Autodesk Inventor part; units mm, degrees
ref_plane "YZ Plane" through (0, 0, 0) normal (1, 0, 0) x (0, 1, 0)
ref_plane "XZ Plane" through (0, 0, 0) normal (0, 1, 0) x (-1, 0, 0)
ref_plane "XY Plane" through (0, 0, 0) normal (0, 0, 1) x (1, 0, 0)
sketch "Sketch1" plane through (0, 0, 0) normal (0, 0, 1) x (1, 0, 0)
  line L0 (-11.35, -6.15) -> (11.35, -6.15) construction
  line L1 (11.35, -6.15) -> (11.35, 6.15) construction
  line L2 (11.35, 6.15) -> (-11.35, 6.15) construction
  line L3 (-11.35, 6.15) -> (-11.35, -6.15) construction
  line L4 (-11.35, -6.15) -> (11.35, 6.15) construction
  line L5 (11.35, -6.15) -> (-11.35, 6.15) construction
  line L6 (-11.5, -6.3) -> (11.5, -6.3)
  line L7 (11.5, -6.3) -> (11.5, 6.3)
  line L8 (11.5, 6.3) -> (-11.5, 6.3)
  line L9 (-11.5, 6.3) -> (-11.5, -6.3)
  line L10 (-11.5, -6.3) -> (11.5, 6.3) construction
  line L11 (11.5, -6.3) -> (-11.5, 6.3) construction
  line L12 (-15.5, -13.1) -> (-15.5, 27.3)
  line L13 (-15.5, 27.3) -> (15.5, 27.3)
  line L14 (15.5, 27.3) -> (15.5, -6.15)
  line L15 (11.5, -6.15) -> (15.5, -6.15)
  line L16 (-11.5, -6.3) -> (-11.5, -9.1)
  line L17 (-11.5, -9.1) -> (14, -9.1)
  line L18 (14, -9.1) -> (14, -13.1)
  line L19 (14, -13.1) -> (-15.5, -13.1)
  circle A0 centre (-14, 0) radius 1.1
  line L20 (-14.9798, 0.5) -> (-15.5, 0.5)
  line L21 (-14.9798, -0.5) -> (-15.5, -0.5)
  line L22 (0, 0) -> (0, 6.3) construction
  circle A1 centre (14, 0) radius 1.1
  line L23 (14.9798, 0.5) -> (15.5, 0.5)
  line L24 (14.9798, -0.5) -> (15.5, -0.5)
  point P0 (15.5, -0.5)
  point P1 (15.5, 0.5)
  point P2 (14, -11.1)
  dimension "d0" = 22.7
  dimension "d1" = 12.3
  dimension "d2" = 0.15
  dimension "d3" = 0.15
  dimension "d5" = 2.95
  dimension "d6" = 4
  dimension "d7" = 21
  dimension "d8" = 4
  dimension "d9" = 4
  dimension "d13" = 2.2
  dimension "d14" = 14
  dimension "d15" = 1
extrude "Extrusion2" add sketch "Sketch1" along normal blind 3 contours L16 L17 L18 L19 L12 L21 A0 L20 L13 L14 L23 A1 L24 L15 L7 L8 L9
sketch "Sketch2" plane through (0, 0, 3) normal (0, 0, 1) x (1, 0, 0)
  line L0 (15.5, 27.3) -> (-15.5, 27.3)
  line L1 (-11.5, 6.3) -> (11.5, 6.3)
  line L2 (10.525, 27.3) -> (13.025, 27.3)
  line L3 (13.025, 27.3) -> (13.025, 19.3)
  line L4 (13.025, 19.3) -> (10.525, 19.3)
  line L5 (10.525, 19.3) -> (10.525, 27.3)
  line L6 (11.5, 6.3) -> (11.5, -6.15)
  line L7 (2.175, 27.3) -> (4.175, 27.3)
  line L8 (4.175, 27.3) -> (4.175, 19.3)
  line L9 (4.175, 19.3) -> (2.175, 19.3)
  line L10 (2.175, 19.3) -> (2.175, 27.3)
  line L11 (14, -9.1) -> (-11.5, -9.1)
  line L12 (-15.5, -13.1) -> (14, -13.1)
  line L13 (10.525, -9.1) -> (13.025, -9.1)
  line L14 (13.025, -9.1) -> (13.025, -13.1)
  line L15 (13.025, -13.1) -> (10.525, -13.1)
  line L16 (10.525, -13.1) -> (10.525, -9.1)
  line L17 (4.175, -9.1) -> (2.175, -9.1)
  line L18 (2.175, -9.1) -> (2.175, -13.1)
  line L19 (2.175, -13.1) -> (4.175, -13.1)
  line L20 (4.175, -13.1) -> (4.175, -9.1)
  point P0 (0, 0)
  point P1 (7.65, 6.55)
  point P2 (7.65, 6.55)
  point P3 (-1.7, 6.55)
  point P4 (10.525, -13.1)
  point P5 (4.175, -13.1)
  point P6 (2.175, -9.1)
  point P7 (10.525, -13.1)
  dimension "d19" = 2.5
  dimension "d22" = 0.975
  dimension "d23" = 2
  dimension "d24" = 6.35
  dimension "d25" = 13
extrude "Extrusion3" add sketch "Sketch2" along normal blind 13.4 contours L3 L4 L5 L0 | L8 L9 L10 L0
sketch "Sketch3" plane through (-15.5, 27.3, 0) normal (0, 1, 0) x (1, 0, 0)
  line L0 (19.675, -3) -> (19.675, -16.4)
  line L1 (26.025, -3) -> (26.025, -16.4)
  line L2 (28.525, -16.4) -> (26.025, -16.4)
  line L3 (17.675, -16.4) -> (19.675, -16.4)
  line L4 (19.675, -16.4) -> (19.675, -19)
  line L5 (19.675, -19) -> (26.025, -19)
  line L6 (26.025, -19) -> (26.025, -16.4)
  line L7 (26.025, -3) -> (19.675, -3)
  line L8 (17.675, -16.4) -> (17.675, -21)
  line L9 (17.675, -21) -> (28.525, -21)
  line L10 (28.525, -21) -> (28.525, -16.4)
  line L11 (19.675, -16) -> (26.025, -16)
  line L12 (19.675, -14) -> (26.025, -14)
  point P0 (15.5, 0)
  dimension "d27" = 16
  dimension "d28" = 4.6
  dimension "d31" = 3
  dimension "d32" = 2
extrude "Extrusion4" add sketch "Sketch3" against normal blind 8 contours L12 L1 L11 L0 | L4 L5 L6 L2 L10 L9 L8 L3
equation "\"d2\" = toleranciaServo + margenServo"
equation "\"d3\" = toleranciaServo + margenServo"
equation "\"d5\" = espesorAcrilico + margenAcrilico"
equation "\"d16\" = espesorPieza"
equation "\"d24\" = juegoCremallera + anchoCremallera - toleranciaAcrilico"
equation "\"toleranciaServo\" = 0.1"
equation "\"espesorAcrilico\" = 2.55"
equation "\"margenAcrilico\" = 0.4"
equation "\"margenServo\" = 0.05"
equation "\"largoPatilla\" = 24"
equation "\"espesorPieza\" = 3"
equation "\"anchoCremallera\" = 6.25"
equation "\"toleranciaAcrilico\" = 0.2"
equation "\"juegoCremallera\" = 0.3"
equation "\"distCremallera\" = 1.075"
properties part number "SoporteServo v2"
For this review, take the finished solid that the model builds, in its own axes (mm). A direction names the side the tool comes from. Give positions to 0.01 mm unless a question says otherwise; leave off trailing zeros. Order: outer loops, then holes, each group sorted by start corner. A loop starts at its lowest first (then second) coordinate and runs counter-clockwise, first axis right, second up.
1) Take a section at A-A (y = 0). Give the boundary of the cut face in (x, z), then the cut area to 3 significant figures.
2) Insertion check: pin 1 (3.5 mm diameter, centred on y = 21.5, z = 17, fed in from -X) (3 decimals); pin 2 (0.9 mm diameter, centred on y = 0, z = 2, fed in from +X); pin 3 (12 mm diameter, centred on x = 8, z = 13.5, fed in from -Y). Each pin has a flat end and moves straight along its axis. Give the tip position at first contact, or say it passes through.
3) Take a section at D-D (y = 23.5). Give the boundary of the cut face in (x, z) (3 decimals).
4) Wall thickness on line 1 (Z direction, x = 9.5, y = 25.5); line 2 (X direction, y = 0, z = 1.7); line 3 (Y direction, x = -14, z = 2.3): over which ranges is each line inside the solid? List them lowest first.
5) The part is to be moulded in two halves that separate along Z. For faces 5 (the face through (10.525, 23, 17)), 6 (the face through (13.025, 23, 12)), 7 (the face through (0, 12, 0)), say which applies: released by +Z, released by -Z, zero draft, split by the parting line, or undercut.
6) Take a section at C-C (x = 7). Give the boundary of the cut face in (y, z), then the cut area to 3 significant figures.
7) Take a section at B-B (z = 3.75). Give the boundary of the cut face in (x, y) (3 decimals), then the cut area to 3 significant figures.
8) For faces 1 (the face through (1, -9.1, 1)), 2 (the face through (-11.5, -1, 1)), 3 (the face through (2.175, 23, 12)), 4 (the face through (7, 23, 16)), list the 3-axis set-ups (+Z, -Z, +X, -X, +Y, -Y) from which the entire face can be reached by the end or side of a thin tool; tool diameter is ignored.
Derived:
1. outline: (-12.9, 0) - (-11.5, 0) - (-11.5, 3) - (-12.9, 3) - close; (11.5, 0) - (12.9, 0) - (12.9, 3) - (11.5, 3) - close
1. area: 8.40 mm2
2. pin 1: stops at x = 2.175
2. pin 2: stops at x = 13
2. pin 3: stops at y = 19.3
3. outline: (-15.5, 0) - (15.5, 0) - (15.5, 3) - (13.025, 3) - (13.025, 21) - (2.175, 21) - (2.175, 3) - (-15.5, 3) - close; hole (4.175, 3) - (10.525, 3) - (10.525, 14) - (4.175, 14) - close; hole (4.175, 16) - (10.525, 16) - (10.525, 19) - (4.175, 19) - close
4. line 1: z = 0 to 3, 14 to 16, 19 to 21
4. line 2: x = -12.9 to -11.5, 11.5 to 12.9
4. line 3: y = -13.1 to -1.1, 1.1 to 27.3
5. face 5: undercut
5. face 6: zero draft
5. face 7: released by -Z
6. outline: (-13.1, 0) - (-9.1, 0) - (-9.1, 3) - (-13.1, 3) - close; (6.3, 0) - (27.3, 0) - (27.3, 3) - (6.3, 3) - close; (19.3, 14) - (27.3, 14) - (27.3, 16) - (19.3, 16) - close; (19.3, 19) - (27.3, 19) - (27.3, 21) - (19.3, 21) - close
6. area: 107 mm2
7. outline: (2.175, 19.3) - (4.175, 19.3) - (4.175, 27.3) - (2.175, 27.3) - close; (10.525, 19.3) - (13.025, 19.3) - (13.025, 27.3) - (10.525, 27.3) - close
7. area: 36.0 mm2
8. face 1: +Z, -Z, +X
8. face 2: +Z, -Z
8. face 3: +Z, -X, +Y, -Y
8. face 4: +Y, -Y
